Autodesk Inventor part; units mm, degrees
ref_plane "YZ Plane" through (0, 0, 0) normal (1, 0, 0) x (0, 1, 0)
ref_plane "XZ Plane" through (0, 0, 0) normal (0, 1, 0) x (-1, 0, 0)
ref_plane "XY Plane" through (0, 0, 0) normal (0, 0, 1) x (1, 0, 0)
sketch "Sketch1" plane through (0, 0, 0) normal (0, 1, 0) x (-1, 0, 0)
  line L0 (-56.25, 58.25) -> (56.25, 58.25)
  line L1 (56.25, 58.25) -> (56.25, -58.25)
  line L2 (56.25, -58.25) -> (-56.25, -58.25)
  line L3 (-56.25, -58.25) -> (-56.25, 58.25)
  line L4 (-56.25, 58.25) -> (56.25, -58.25) construction
  line L5 (56.25, 58.25) -> (-56.25, -58.25) construction
  point P0 (0, 0)
  dimension "d0" = 112.5
  dimension "d1" = 116.5
extrude "Extrusion1" add sketch "Sketch1" along normal blind 5
sketch "Sketch2" plane through (0, 5, 0) normal (0, 1, 0) x (1, 0, 0)
  circle A0 centre (18.5, 28) radius 23.85
  circle A1 centre (37, -23.25) radius 13.85
  circle A2 centre (-35, -38.75) radius 13.85
  circle A3 centre (-30.9, 25.8) radius 13.85
  circle A4 centre (0, -23.25) radius 13.85
  line L0 (56.25, 58.25) -> (-56.25, 58.25)
  line L1 (-56.25, -58.25) -> (56.25, -58.25)
  line L2 (0, -105.9299) -> (0, 123.2086) construction
  line L3 (-76.4777, -38.75) -> (-5.35, -38.75) construction
  line L4 (-123.5447, -23.25) -> (82.5572, -23.25) construction
  line L5 (56.25, -58.25) -> (56.25, 58.25) construction
  point P0 (0, 0)
  dimension "d4" = 47.7
  dimension "d5" = 27.7
  dimension "d6" = 27.7
  dimension "d7" = 27.7
  dimension "d8" = 27.7
  dimension "d9" = 116.5
  dimension "d10" = 112.5
  dimension "d13" = 37
  dimension "d14" = 18.5
  dimension "d15" = 30.9
  dimension "d18" = 19.5
  dimension "d19" = 35
  dimension "d20" = 35
  dimension "d42" = 25.8
  dimension "d43" = 28
extrude "Extrusion2" cut sketch "Sketch2" against normal blind 5
sketch "Sketch5" plane through (0, 5, 0) normal (0, 1, 0) x (1, 0, 0)
  line L0 (-56.25, 58.25) -> (-56.25, -58.25) construction
  circle A0 centre (0, -23.25) radius 13.85 construction
  circle A1 centre (37, -23.25) radius 13.85 construction
  circle A2 centre (-30.9, 25.8) radius 13.85 construction
  line L1 (56.25, 58.25) -> (-56.25, 58.25) construction
  line L2 (-17.15, -23.25) -> (-13.85, -23.25) construction
  line L3 (-46.75, -8.1822) -> (-46.85, -8.1822)
  line L4 (-13.85, -23.25) -> (-17.15, -23.25)
  line L5 (56.25, -58.25) -> (56.25, 58.25)
  line L6 (-46.85, -8.1822) -> (-46.75, -8.1822)
  arc A3 (-13.85, -23.25) -> (13.85, -23.25) centre (0, -23.25) ccw
  arc A4 (23.15, -23.25) -> (50.85, -23.25) centre (37, -23.25) ccw
  line L7 (-44.75, 58.25) -> (42.35, 58.25)
  line L8 (-48.85, -38.75) -> (-48.85, -38.75)
  line L9 (-50.85, -36.75) -> (-50.85, -10.1822)
  line L10 (-48.85, -8.1822) -> (-48.75, -8.1822)
  arc A5 (-50.85, -36.75) -> (-48.85, -38.75) centre (-48.85, -36.75) ccw
  arc A6 (-48.85, -8.1822) -> (-50.85, -10.1822) centre (-48.85, -10.1822) ccw
  line L11 (50.85, -23.25) -> (50.85, -23.25)
  line L12 (52.85, -21.25) -> (52.85, -4.75)
  line L13 (50.85, -2.75) -> (46.35, -2.75)
  arc A7 (50.85, -23.25) -> (52.85, -21.25) centre (50.85, -21.25) ccw
  arc A8 (52.85, -4.75) -> (50.85, -2.75) centre (50.85, -4.75) ccw
  line L14 (-44.7516, 25.8) -> (-44.7516, 25.8)
  line L15 (-46.75, 28.0339) -> (-46.75, 58.25)
  line L16 (-44.75, 58.25) -> (-46.75, 58.25)
  line L17 (-17.0566, 26.2282) -> (-17.0566, 26.2282)
  line L18 (-15.05, 27.8) -> (-15.05, 42.25)
  line L19 (-5.35, 27.98) -> (-5.35, 27.98)
  line L20 (-7.35, 30.25) -> (-7.35, 42.25)
  line L21 (42.35, 27.98) -> (42.35, 27.98)
  line L22 (44.35, 58.25) -> (42.35, 58.25)
  circle A9 centre (0, -23.25) radius 13.85
  circle A10 centre (37, -23.25) radius 13.85
  line L23 (44.35, 58.25) -> (44.35, -0.75)
  line L24 (42.35, 27.98) -> (44.35, 27.98)
  line L25 (-5.35, 27.98) -> (-5.35, 27.98)
  line L26 (-7.35, 29.98) -> (-7.35, 30.25)
  line L27 (-17.0566, 26.2282) -> (-17.0566, 26.2282)
  line L28 (-15.05, 28.0029) -> (-15.05, 28.0029)
  line L29 (-46.75, 28.0339) -> (-46.75, -6.1822)
  arc A11 (-48.75, -8.1822) -> (-46.75, -6.1822) centre (-48.75, -6.1822) ccw
  line L30 (-44.75, 25.8) -> (-46.75, 25.8)
  line L31 (-21.15, -38.75) -> (-21.15, -38.75)
  line L32 (-19.15, -36.75) -> (-19.15, -25.25)
  arc A12 (-21.15, -38.75) -> (-19.15, -36.75) centre (-21.15, -36.75) ccw
  arc A13 (-17.15, -23.25) -> (-19.15, -25.25) centre (-17.15, -25.25) ccw
  line L33 (-17.05, 25.8) -> (-17.05, 25.8)
  arc A14 (-17.05, 25.8) -> (-15.05, 27.8) centre (-17.05, 27.8) ccw
  line L34 (-56.25, -58.25) -> (56.25, -58.25)
  line L35 (56.25, -58.25) -> (56.25, 58.25)
  line L36 (56.25, 58.25) -> (-56.25, 58.25)
  line L37 (-56.25, 58.25) -> (-56.25, -58.25)
  circle A15 centre (-30.9, 25.8) radius 13.85
  circle A16 centre (-30.9, 25.8) radius 13.85
  line L38 (13.85, -23.25) -> (13.85, -13.25)
  circle A17 centre (0, -23.25) radius 13.85
  line L39 (23.15, -23.25) -> (23.15, -13.25)
  circle A18 centre (37, -23.25) radius 13.85
  arc A19 (23.15, -13.25) -> (13.85, -13.25) centre (18.5, -13.25) ccw
  circle A20 centre (18.5, 28) radius 23.85
  circle A21 centre (18.5, 28) radius 23.85
  line L40 (56.25, 58.25) -> (-56.25, 58.25)
  circle A22 centre (-35, -38.75) radius 13.85
  circle A23 centre (-35, -38.75) radius 13.85
  arc A24 (44.35, -0.75) -> (46.35, -2.75) centre (46.35, -0.75) ccw
  line L41 (-5.35, 27.98) -> (-5.35, 27.98)
  arc A25 (-7.35, 29.98) -> (-5.35, 27.98) centre (-5.35, 29.98) ccw
  line L42 (-13.05, 44.25) -> (-9.35, 44.25)
  arc A26 (-13.05, 44.25) -> (-15.05, 42.25) centre (-13.05, 42.25) ccw
  arc A27 (-7.35, 42.25) -> (-9.35, 44.25) centre (-9.35, 42.25) ccw
  point P0 (0, 0)
  point P1 (0, 0)
  point P2 (44.35, -2.75)
  point P3 (-50.85, -38.75)
  point P4 (52.85, -23.25)
  point P5 (-15.05, 58.25)
  point P6 (-7.35, 58.25)
  point P7 (-48.85, -40.25)
  point P8 (50.85, -23.25)
  point P9 (-21.15, -40.25)
  point P10 (50.85, -23.25)
  point P11 (-7.35, 58.25)
  point P12 (50.85, -23.25)
  point P13 (-17.05, 25.8)
  point P14 (-7.35, 27.98)
  point P15 (-7.35, 29.98)
  point P16 (-21.15, -38.75)
  point P17 (-48.85, -38.75)
  dimension "d53" = 27.7
  dimension "d54" = 27.7
  dimension "d26" = 2
  dimension "d27" = 2
  dimension "d28" = 2
  dimension "d29" = 2
  dimension "d30" = 2
  dimension "d32" = 2
  dimension "d33" = 2
  dimension "d34" = 2
  dimension "d35" = 2
  dimension "d38" = 27.7
  dimension "d39" = 10
  dimension "d40" = 10
  dimension "d45" = 25.8
  dimension "d46" = 23.25
  dimension "d47" = 23.25
  dimension "d50" = 37
  dimension "d56" = 19.15
  dimension "d57" = 50.85
  dimension "d58" = 46.75
  dimension "d59" = 2
  dimension "d60" = 6.1822
  dimension "d61" = 31.7
  dimension "d63" = 30.9
  dimension "d64" = 3.4
  dimension "d65" = 11.9
  dimension "d66" = 61
  dimension "d67" = 47.7
  dimension "d68" = 28
  dimension "d69" = 18.5
  dimension "d71" = 30.27
  dimension "d72" = 27.7
  dimension "d73" = 2
  dimension "d74" = 30.27
  dimension "d75" = 2
  dimension "d76" = 112.5
  dimension "d77" = 116.5
  dimension "d79" = 14
  dimension "d80" = 2
  dimension "d81" = 51.7
  dimension "d82" = 2
extrude "Extrusion3" cut sketch "Sketch5" against normal blind 10 contours A3 L38 A19 L39 A4 A7 L12 A8 L13 A24 L23 L36 L5 L34 L37 L15 L29 A11 L10 A6 L9 A5 A22 A12 L32 A13 L4 | L29 L15 L16 L7 L22 L23 L24 A20 A25 L26 L20 A27 L42 A26 L18 A14 A15 L30
fillet "Fillet2" radius 1 2 edges at (13.85, 2.5, 23.25) (23.15, 2.5, 23.25)
sketch "Sketch7" plane through (0, 5, 0) normal (0, 1, 0) x (1, 0, 0)
  line L0 (-7.35, 29.98) -> (-7.35, 42.25)
  line L1 (-9.35, 44.25) -> (-13.05, 44.25)
  point P0 (0, 0)
  point P1 (-34, -13)
  point P2 (-13, 11)
  point P3 (36, -2)
  point P4 (-11.2, 39.75)
  dimension "d83" = 13
  dimension "d84" = 34
  dimension "d85" = 36
  dimension "d86" = 2
  dimension "d87" = 11
  dimension "d88" = 13
  dimension "d96" = 3.85
  dimension "d97" = 4.5
hole "Hole1" at (-34, 5, 13) at (-13, 5, -11) at (36, 5, 2) direction (0, -1, 0) diameter 3.8 end through all
hole "Hole2" at (-11.2, 5, -39.75) direction (0, -1, 0) diameter 4.2 end through all
properties part number "Bottle layout pt2"
CAD build for the part. Positions are in the model's coordinates, mm. A direction names the side the tool comes from. Round coordinates to 2 decimals unless told otherwise and drop trailing zeros. Order: outer loops, then holes, each group sorted by start corner. A loop starts at its lowest first (then second) coordinate and runs counter-clockwise, first axis right, second up. Notation, with made-up numbers: (-26, -13) - (27, -13) arc R32 cw to (27, 16) - close; hole circle Ø10 at (19, 81.5). An arc over 180 degrees is marked (long way). Answer in a Markdown table with one row per item. Add a question column.
(1) 3-axis set-ups, long thin cutter, end or side, ignore diameter. For faces 5 (the face through (44.35, 3, -14)), 6 (the face through (-19.15, 3, 31)), 7 (the face through (23.15, 3, 15)), 8 (the face through (-50.85, 3, 24)): which of +Z, -Z, +X, -X, +Y, -Y reach the whole face in a straight line?
(2) Band-saw the part on B-B on x = 36. List the corners of the cut face in (y, z), and give its area (3 significant figures).
(3) Band-saw the part on D-D on y = 1.25. Count the separate pieces of the cut face and the enclosed holes in it, and give its area (3 significant figures).
(4) Drop flat-ended pins along their axis: pin 1 Ø0.6 at (x, y) = (44, 3) entering from -Z; pin 2 Ø0.6 at (x, y) = (-45.5, 2) entering from -Z; pin 3 Ø3 at (y, z) = (1, 26.5) entering from +X. Give the stop position or say it passes through.
(5) Probe L1, parallel to X at y = 2.55, z = -22.5; L2, parallel to X at y = 1.15, z = 2; L3, parallel to X at y = 2.2, z = -11. List the from-to ranges inside material, lowest first. Write a range as [from, to].
(6) Band-saw the part on A-A on z = -39.75. List the corners of the cut face in (x, y).
(7) Band-saw the part on C-C on x = 18.5. List the corners of the cut face in (y, z), and give its area (4 significant figures).
(8) Mould opens along X. For faces 1 (the face through (52.28, 2.54, 3.35)), 2 (the face through (-15, 3, 23.25)), 3 (the face through (-15.05, 3, -35)), 4 (the face through (18.6, 2.5, 8.6)) say: +X half, -X half, draft (parallel to the pull), parting line (faces both ways), or undercut.
Data:
| question | item | result |
|---|---|---|
| 1 | face 5 | -Z, +X, +Y, -Y |
| 1 | face 6 | +Z, +X, +Y, -Y |
| 1 | face 7 | +Z, +Y, -Y |
| 1 | face 8 | +Z, -Z, -X, +Y, -Y |
| 2 | outline | (0, -11.8) - (5, -11.8) - (5, 0.1) - (0, 0.1) - close; (0, 3.9) - (5, 3.9) - (5, 9.44) - (0, 9.44) - close |
| 2 | area | 87.2 mm^2 |
| 3 | separate pieces | 1 |
| 3 | enclosed holes | 4 |
| 3 | area | 3,170 mm^2 |
| 4 | pin 1 | stops at z = -27.98 |
| 4 | pin 2 | stops at z = -25.8 |
| 4 | pin 3 | stops at x = -19.13 |
| 5 | L1 | x = [-46.75, -44.35], [-17.45, -4.71], [41.71, 44.35] |
| 5 | L2 | x = [-46.75, 34.1], [37.9, 44.79] |
| 5 | L3 | x = [-46.75, -14.9], [-11.1, 1.77], [35.23, 44.35] |
| 6 | outline | (-15.05, 0) - (-13.3, 0) - (-13.3, 5) - (-15.05, 5) - close; (-9.1, 0) - (-7.35, 0) - (-7.35, 5) - (-9.1, 5) - close |
| 7 | outline | (0, -4.15) - (5, -4.15) - (5, 8.6) - (0, 8.6) - close |
| 7 | area | 63.75 mm^2 |
| 8 | face 1 | +X half |
| 8 | face 2 | draft |
| 8 | face 3 | -X half |
| 8 | face 4 | undercut |
